Here's how the part is built. I have some questions about the finished solid (model axes, mm). Coordinates: 2 decimals unless noted, no trailing zeros. Order: outer loops, then holes, each group sorted by start corner. A loop starts at its lowest first (then second) coordinate and runs counter-clockwise, first axis right, second up. Notation, with made-up numbers: (-26, 50.5) - (18, 50.5) arc R21 cw to (18, 57.5) - close; hole circle Ø10 at (25.25, 50.25). An arc over 180 degrees is marked (long way). Answer as CSV lines item,"result". Start each with the question number.
Q1. Suppose I cut it at C-C (y = -3.5). Please give me the cut outline in (x, z).
Q2. Suppose I cut it at A-A (x = -30.5). Please give me the cut outline in (y, z).
Q3. For pin 1 Ø1.9 at (x, y) = (0, 3.5) entering from -Z, with a flat end and sliding along its axis, tell me the tip position at first contact or that it passes through.
Q4. Thinking about a two-plate mould opening in Y: for faces 1 (the face through (29.39, -3.96, -0.01)), 2 (the face through (22.7, 3.55, -0.01)), 3 (the face through (-1, 0, 0.5)), which applies, released by +Y, released by -Y, zero draft, split by the parting line, or undercut?
Q5. Suppose I cut it at B-B (z = -0.05). Please give me the cut outline in (x, y).
Q6. I need wall thicknesses on line 1 (X direction, y = -2.5, z = 0.4); line 2 (Y direction, x = 30.5, z = 0.2); line 3 (Y direction, x = 21.5, z = 0.25). Which ranges of each line are inside material? Lowest first, please.
from build123d import *

# Parameters (mm, degrees)
SKETCH1_W           = 81
SKETCH1_H           = 12
BOSS_EXTRUDE1_DEPTH = 0.5
M2_HOLE1_AD_D       = 2.4
M2_HOLE1_AD_DEPTH   = 100
M2_HOLE1_AD_TIP     = 0.721032743
M2_HOLE2_AD_D       = 2.4
M2_HOLE2_AD_DEPTH   = 100
M2_HOLE2_AD_TIP     = 0.721032743
M2_HOLE3_AE_D       = 2.4
M2_HOLE3_AE_DEPTH   = 200
M2_HOLE3_AE_TIP     = 0.721032743
FILLET1_R           = 0.1


with BuildPart() as part:
    # Sketch1 → Boss-Extrude1 (new, symmetric)
    with BuildSketch(Plane.XY):
        Rectangle(SKETCH1_W, SKETCH1_H)
    extrude(amount=BOSS_EXTRUDE1_DEPTH, both=True)

    # M2 Hole1 - AD
    with Locations(Plane.XY.offset(0.5)):
        with Locations((-30.5, -3.5), (30.5, -3.5)):
            Hole(M2_HOLE1_AD_D / 2, depth=M2_HOLE1_AD_DEPTH)
            with Locations((0, 0, -(M2_HOLE1_AD_DEPTH + M2_HOLE1_AD_TIP / 2))):  # 118° drill point
                Cone(0, M2_HOLE1_AD_D / 2, M2_HOLE1_AD_TIP, mode=Mode.SUBTRACT)

    # M2 Hole2 - AD
    with Locations(Plane.XY.offset(0.5)):
        with Locations((-21.5, 3.5), (21.5, 3.5)):
            Hole(M2_HOLE2_AD_D / 2, depth=M2_HOLE2_AD_DEPTH)
            with Locations((0, 0, -(M2_HOLE2_AD_DEPTH + M2_HOLE2_AD_TIP / 2))):  # 118° drill point
                Cone(0, M2_HOLE2_AD_D / 2, M2_HOLE2_AD_TIP, mode=Mode.SUBTRACT)

    # M2 Hole3 - AE
    with Locations(Plane.XY.offset(0.5)):
        with Locations((0, 3.5)):
            Hole(M2_HOLE3_AE_D / 2, depth=M2_HOLE3_AE_DEPTH)
            with Locations((0, 0, -(M2_HOLE3_AE_DEPTH + M2_HOLE3_AE_TIP / 2))):  # 118° drill point
                Cone(0, M2_HOLE3_AE_D / 2, M2_HOLE3_AE_TIP, mode=Mode.SUBTRACT)

    # Fillet1
    fillet1_edges = [part.edges().sort_by_distance(p)[0] for p in [
        (-40.5, 0, 0.5),
        (40.5, 0, 0.5),
        (-40.5, 0, -0.5),
        (40.5, 0, -0.5),
    ]]
    fillet(fillet1_edges, radius=FILLET1_R)


solid = part.part
Here are the results:
1,outline,"(-40.5, -0.4) arc R0.1 ccw to (-40.4, -0.5) - (-31.7, -0.5) - (-31.7, 0.5) - (-40.4, 0.5) arc R0.1 ccw to (-40.5, 0.4) - close; (-29.3, -0.5) - (29.3, -0.5) - (29.3, 0.5) - (-29.3, 0.5) - close; (31.7, -0.5) - (40.4, -0.5) arc R0.1 ccw to (40.5, -0.4) - (40.5, 0.4) arc R0.1 ccw to (40.4, 0.5) - (31.7, 0.5) - close"
2,outline,"(-6, -0.5) - (-4.7, -0.5) - (-4.7, 0.5) - (-6, 0.5) - close; (-2.3, -0.5) - (6, -0.5) - (6, 0.5) - (-2.3, 0.5) - close"
3,pin 1,"passes through"
4,face 1,"undercut"
4,face 2,"undercut"
4,face 3,"zero draft"
5,outline,"(-40.5, -6) - (40.5, -6) - (40.5, 6) - (-40.5, 6) - close; hole circle Ø2.4 at (-30.5, -3.5); hole circle Ø2.4 at (-21.5, 3.5); hole circle Ø2.4 at (0, 3.5); hole circle Ø2.4 at (21.5, 3.5); hole circle Ø2.4 at (30.5, -3.5)"
6,line 1,"x = -40.5 to -31.16, -29.84 to 29.84, 31.16 to 40.5"
6,line 2,"y = -6 to -4.7, -2.3 to 6"
6,line 3,"y = -6 to 2.3, 4.7 to 6"
